Check sheet for the modelled part. Datum: model origin and axes. Units: mm. Coordinates: 2 decimals unless noted, no trailing zeros. Write each loop counter-clockwise with the first axis right and the second up, starting at its lowest first coordinate (ties: lowest second). Pieces come first, ordered by that corner, then holes. Notation, with made-up numbers: (70, 5) -> (92, 5) arc R20 cw to (92, 39) -> close; hole circle Ø8 at (-11, 22). An arc over 180 degrees is marked (long way). One line per item, written item: value. Start each with the question number.
1) Draft check along X on faces 1 (the flat face through (7.5, 1, 0)), 2 (the cylindrical face through (5.36, 1.01, -0.59)), 3 (the flat face through (0, 1, -7.5)). Enter one of: +X half, -X half, draft (parallel to the pull), parting line (faces both ways), or undercut.
2) Sectioned sample at C-C on y = 1.1. Enter the section's corners in (x, z).
3) Sectioned sample at D-D on x = -4.5. Enter the section's corners in (y, z), plus the area to 3 significant figures.
4) Sectioned sample at B-B on x = 3.5. Enter the section's corners in (y, z).
5) Gauge pin test, flat end, axial feed: P1, Ø1.5, axis at x = -4.5, z = -2, coming from the -Y side. Record the tip position at first contact, or that the pin passes through.
6) Sectioned sample at A-A on z = 0. Enter the section's corners in (x, y).
7) Scan lines: line 1 along Z through (x, y) = (-4.5, 1.15); line 2 along Z through (x, y) = (3.5, 0.9); line 3 along Z through (x, y) = (-3.75, 1.6). Record each from-to range of solid material in increasing order. Write a range as [from, to].
```python
from build123d import *

# Parameters (mm, degrees)
SKETCH2_W           = 15
SKETCH2_H           = 15
BOSS_EXTRUDE1_DEPTH = 2
SKETCH3_R           = 0.95
CUT_EXTRUDE1_DEPTH  = 2
SKETCH4_R           = 1.95
CUT_EXTRUDE2_DEPTH  = 2


with BuildPart() as part:
    # Sketch2 → Boss-Extrude1 (new body)
    with BuildSketch(Plane(origin=(0, 0, 0), x_dir=(1, 0, 0), z_dir=(0, 1, 0))):
        Rectangle(SKETCH2_W, SKETCH2_H)
    extrude(amount=BOSS_EXTRUDE1_DEPTH)

    # Sketch3 → Cut-Extrude1 (cut)
    with BuildSketch(Plane(origin=(0, 2, 0), x_dir=(1, 0, 0), z_dir=(0, 1, 0))):
        with Locations((-4.5, -2)):
            Circle(SKETCH3_R)
        with Locations((-4.5, 2)):
            Circle(SKETCH3_R)
    extrude(amount=-CUT_EXTRUDE1_DEPTH, mode=Mode.SUBTRACT)

    # Sketch4 → Cut-Extrude2 (cut)
    with BuildSketch(Plane(origin=(0, 2, 0), x_dir=(1, 0, 0), z_dir=(0, 1, 0))):
        with Locations((3.5, 0)):
            Circle(SKETCH4_R)
    extrude(amount=-CUT_EXTRUDE2_DEPTH, mode=Mode.SUBTRACT)


solid = part.part
```
Answers:
1. face 1: +X half
1. face 2: undercut
1. face 3: draft
2. outline: (-7.5, -7.5) -> (7.5, -7.5) -> (7.5, 7.5) -> (-7.5, 7.5) -> close; hole circle Ø1.9 at (-4.5, -2); hole circle Ø1.9 at (-4.5, 2); hole circle Ø3.9 at (3.5, 0)
3. outline: (0, -7.5) -> (2, -7.5) -> (2, -2.95) -> (0, -2.95) -> close; (0, -1.05) -> (2, -1.05) -> (2, 1.05) -> (0, 1.05) -> close; (0, 2.95) -> (2, 2.95) -> (2, 7.5) -> (0, 7.5) -> close
3. area: 22.4 mm2
4. outline: (0, -7.5) -> (2, -7.5) -> (2, -1.95) -> (0, -1.95) -> close; (0, 1.95) -> (2, 1.95) -> (2, 7.5) -> (0, 7.5) -> close
5. P1: passes through
6. outline: (-7.5, 0) -> (1.55, 0) -> (1.55, 2) -> (-7.5, 2) -> close; (5.45, 0) -> (7.5, 0) -> (7.5, 2) -> (5.45, 2) -> close
7. line 1: z = [-7.5, -2.95], [-1.05, 1.05], [2.95, 7.5]
7. line 2: z = [-7.5, -1.95], [1.95, 7.5]
7. line 3: z = [-7.5, -2.58], [-1.42, 1.42], [2.58, 7.5]
